The model under review builds one solid part; all positions refer to its coordinate system, in mm. Give positions to 0.01 mm unless a question says otherwise; leave off trailing zeros. Order: outer loops, then holes, each group sorted by start corner. A loop starts at its lowest first (then second) coordinate and runs counter-clockwise, first axis right, second up. Notation, with made-up numbers: (16.25, 66) - (31.25, 66) arc R34 cw to (31.25, 99) - close; hole circle Ø5 at (-19.75, -8.75). An arc over 180 degrees is marked (long way). Write item = value, one per line. Start each with the question number.
1. We need section B-B, the plane x = -3.81. Give the boundary of the cut face in (y, z).
2. We need section D-D, the plane z = -18.25. Give the boundary of the cut face in (x, y).
3. We need section C-C, the plane y = 0.2. State how many separate pieces and enclosed holes the cut face has, and give its area (3 significant figures).
4. Wall thickness on probe 1 along Z at (x, y) = (6, 0.25); probe 2 along Z at (x, y) = (-3.5, 0.2); probe 3 along X at (y, z) = (0.2, -19.25): over which ranges is each line inside the solid? List them lowest first.
5. We need section A-A, the plane x = 15.24. Give the boundary of the cut face in (y, z), and give its area (3 significant figures).
from build123d import *

# Parameters (mm, degrees)
SKETCH2_R               = 25.4
BOSS_EXTRUDE1_DEPTH     = 0.508
SKETCH3_R               = 1.016
CUT_EXTRUDE2_DEPTH      = 36.924616407
FILL_PATTERN1_OUTLINE_R = 1.016
FILL_PATTERN1_DEPTH     = 0.508
SKETCH7_W               = 63.5
SKETCH7_H               = 31.75
CUT_EXTRUDE5_DEPTH      = 36.924616407


# Read off the part's stored shape, not the designer's step: Fill Pattern1
with BuildPart() as part:
    # Sketch2 → Boss-Extrude1 (new body)
    with BuildSketch(Plane(origin=(0, 0, 0), x_dir=(1, 0, 0), z_dir=(0, 1, 0))):
        with Locations(Location((0, 0, 0), (0, 0, 270))):
            Circle(SKETCH2_R)
    extrude(amount=BOSS_EXTRUDE1_DEPTH)

    # Sketch3 → Cut-Extrude2 (cut, through all)
    with BuildSketch(Plane(origin=(0, 0.508, 0), x_dir=(1, 0, 0), z_dir=(0, 1, 0))):
        with Locations(Location((0, 0, 0), (0, 0, 270))):
            Circle(SKETCH3_R)
    extrude(amount=-CUT_EXTRUDE2_DEPTH, mode=Mode.SUBTRACT)

    # Fill Pattern1 outline → Fill Pattern1 (cut)
    with BuildSketch(Plane(origin=(0, 0, 0), x_dir=(1, 0, 0), z_dir=(0, 1, 0))):
        with Locations((20.955, -3.299556788)):
            Circle(FILL_PATTERN1_OUTLINE_R)
        with Locations((-11.43, -6.599113577)):
            Circle(FILL_PATTERN1_OUTLINE_R)
        with Locations((-13.335, -9.898670365)):
            Circle(FILL_PATTERN1_OUTLINE_R)
        with Locations((-15.24, -13.198227154)):
            Circle(FILL_PATTERN1_OUTLINE_R)
        with Locations((0, 19.797340731)):
            Circle(FILL_PATTERN1_OUTLINE_R)
        with Locations((-9.525, -3.299556788)):
            Circle(FILL_PATTERN1_OUTLINE_R)
        with Locations((-7.62, 0)):
            Circle(FILL_PATTERN1_OUTLINE_R)
        with Locations((-5.715, 3.299556788)):
            Circle(FILL_PATTERN1_OUTLINE_R)
        with Locations((-3.81, 6.599113577)):
            Circle(FILL_PATTERN1_OUTLINE_R)
        with Locations((-1.905, 16.497783942)):
            Circle(FILL_PATTERN1_OUTLINE_R)
        with Locations((-3.81, 13.198227154)):
            Circle(FILL_PATTERN1_OUTLINE_R)
        with Locations((-5.715, 9.898670365)):
            Circle(FILL_PATTERN1_OUTLINE_R)
        with Locations((-7.62, 6.599113577)):
            Circle(FILL_PATTERN1_OUTLINE_R)
        with Locations((-9.525, 3.299556788)):
            Circle(FILL_PATTERN1_OUTLINE_R)
        with Locations((-11.43, 0)):
            Circle(FILL_PATTERN1_OUTLINE_R)
        with Locations((-13.335, -3.299556788)):
            Circle(FILL_PATTERN1_OUTLINE_R)
        with Locations((-15.24, -6.599113577)):
            Circle(FILL_PATTERN1_OUTLINE_R)
        with Locations((7.62, 19.797340731)):
            Circle(FILL_PATTERN1_OUTLINE_R)
        with Locations((5.715, 16.497783942)):
            Circle(FILL_PATTERN1_OUTLINE_R)
        with Locations((3.81, 13.198227154)):
            Circle(FILL_PATTERN1_OUTLINE_R)
        with Locations((1.905, 9.898670365)):
            Circle(FILL_PATTERN1_OUTLINE_R)
        with Locations((0, 6.599113577)):
            Circle(FILL_PATTERN1_OUTLINE_R)
        with Locations((-1.905, 3.299556788)):
            Circle(FILL_PATTERN1_OUTLINE_R)
        with Locations((-3.81, 0)):
            Circle(FILL_PATTERN1_OUTLINE_R)
        with Locations((-5.715, -3.299556788)):
            Circle(FILL_PATTERN1_OUTLINE_R)
        with Locations((-7.62, -6.599113577)):
            Circle(FILL_PATTERN1_OUTLINE_R)
        with Locations((-9.525, -9.898670365)):
            Circle(FILL_PATTERN1_OUTLINE_R)
        with Locations((-11.43, -13.198227154)):
            Circle(FILL_PATTERN1_OUTLINE_R)
        with Locations((-13.335, -16.497783942)):
            Circle(FILL_PATTERN1_OUTLINE_R)
        with Locations((3.81, 19.797340731)):
            Circle(FILL_PATTERN1_OUTLINE_R)
        with Locations((1.905, 16.497783942)):
            Circle(FILL_PATTERN1_OUTLINE_R)
        with Locations((0, 13.198227154)):
            Circle(FILL_PATTERN1_OUTLINE_R)
        with Locations((-1.905, 9.898670365)):
            Circle(FILL_PATTERN1_OUTLINE_R)
        with Locations((-19.05, 0)):
            Circle(FILL_PATTERN1_OUTLINE_R)
        with Locations((-20.955, -3.299556788)):
            Circle(FILL_PATTERN1_OUTLINE_R)
        with Locations((-13.335, 16.497783942)):
            Circle(FILL_PATTERN1_OUTLINE_R)
        with Locations((-15.24, 13.198227154)):
            Circle(FILL_PATTERN1_OUTLINE_R)
        with Locations((-17.145, 9.898670365)):
            Circle(FILL_PATTERN1_OUTLINE_R)
        with Locations((-19.05, 6.599113577)):
            Circle(FILL_PATTERN1_OUTLINE_R)
        with Locations((-20.955, 3.299556788)):
            Circle(FILL_PATTERN1_OUTLINE_R)
        with Locations((-15.24, 0)):
            Circle(FILL_PATTERN1_OUTLINE_R)
        with Locations((-13.335, 3.299556788)):
            Circle(FILL_PATTERN1_OUTLINE_R)
        with Locations((-11.43, 6.599113577)):
            Circle(FILL_PATTERN1_OUTLINE_R)
        with Locations((-9.525, 9.898670365)):
            Circle(FILL_PATTERN1_OUTLINE_R)
        with Locations((-17.145, -9.898670365)):
            Circle(FILL_PATTERN1_OUTLINE_R)
        with Locations((-3.81, 19.797340731)):
            Circle(FILL_PATTERN1_OUTLINE_R)
        with Locations((-5.715, 16.497783942)):
            Circle(FILL_PATTERN1_OUTLINE_R)
        with Locations((-7.62, 13.198227154)):
            Circle(FILL_PATTERN1_OUTLINE_R)
        with Locations((-17.145, 3.299556788)):
            Circle(FILL_PATTERN1_OUTLINE_R)
        with Locations((-15.24, 6.599113577)):
            Circle(FILL_PATTERN1_OUTLINE_R)
        with Locations((-13.335, 9.898670365)):
            Circle(FILL_PATTERN1_OUTLINE_R)
        with Locations((-11.43, 13.198227154)):
            Circle(FILL_PATTERN1_OUTLINE_R)
        with Locations((-9.525, 16.497783942)):
            Circle(FILL_PATTERN1_OUTLINE_R)
        with Locations((-7.62, 19.797340731)):
            Circle(FILL_PATTERN1_OUTLINE_R)
        with Locations((-19.05, -6.599113577)):
            Circle(FILL_PATTERN1_OUTLINE_R)
        with Locations((-17.145, -3.299556788)):
            Circle(FILL_PATTERN1_OUTLINE_R)
        with Locations((3.81, -19.797340731)):
            Circle(FILL_PATTERN1_OUTLINE_R)
        with Locations((17.145, 9.898670365)):
            Circle(FILL_PATTERN1_OUTLINE_R)
        with Locations((15.24, 6.599113577)):
            Circle(FILL_PATTERN1_OUTLINE_R)
        with Locations((13.335, 3.299556788)):
            Circle(FILL_PATTERN1_OUTLINE_R)
        with Locations((5.715, -16.497783942)):
            Circle(FILL_PATTERN1_OUTLINE_R)
        with Locations((7.62, -13.198227154)):
            Circle(FILL_PATTERN1_OUTLINE_R)
        with Locations((9.525, -9.898670365)):
            Circle(FILL_PATTERN1_OUTLINE_R)
        with Locations((11.43, -6.599113577)):
            Circle(FILL_PATTERN1_OUTLINE_R)
        with Locations((3.81, -13.198227154)):
            Circle(FILL_PATTERN1_OUTLINE_R)
        with Locations((1.905, -16.497783942)):
            Circle(FILL_PATTERN1_OUTLINE_R)
        with Locations((0, -19.797340731)):
            Circle(FILL_PATTERN1_OUTLINE_R)
        with Locations((15.24, 13.198227154)):
            Circle(FILL_PATTERN1_OUTLINE_R)
        with Locations((5.715, -9.898670365)):
            Circle(FILL_PATTERN1_OUTLINE_R)
        with Locations((7.62, -6.599113577)):
            Circle(FILL_PATTERN1_OUTLINE_R)
        with Locations((9.525, -3.299556788)):
            Circle(FILL_PATTERN1_OUTLINE_R)
        with Locations((11.43, 0)):
            Circle(FILL_PATTERN1_OUTLINE_R)
        with Locations((15.24, -6.599113577)):
            Circle(FILL_PATTERN1_OUTLINE_R)
        with Locations((17.145, -3.299556788)):
            Circle(FILL_PATTERN1_OUTLINE_R)
        with Locations((19.05, 0)):
            Circle(FILL_PATTERN1_OUTLINE_R)
        with Locations((20.955, 3.299556788)):
            Circle(FILL_PATTERN1_OUTLINE_R)
        with Locations((13.335, -16.497783942)):
            Circle(FILL_PATTERN1_OUTLINE_R)
        with Locations((15.24, -13.198227154)):
            Circle(FILL_PATTERN1_OUTLINE_R)
        with Locations((17.145, -9.898670365)):
            Circle(FILL_PATTERN1_OUTLINE_R)
        with Locations((19.05, -6.599113577)):
            Circle(FILL_PATTERN1_OUTLINE_R)
        with Locations((13.335, -9.898670365)):
            Circle(FILL_PATTERN1_OUTLINE_R)
        with Locations((11.43, -13.198227154)):
            Circle(FILL_PATTERN1_OUTLINE_R)
        with Locations((9.525, -16.497783942)):
            Circle(FILL_PATTERN1_OUTLINE_R)
        with Locations((7.62, -19.797340731)):
            Circle(FILL_PATTERN1_OUTLINE_R)
        with Locations((19.05, 6.599113577)):
            Circle(FILL_PATTERN1_OUTLINE_R)
        with Locations((17.145, 3.299556788)):
            Circle(FILL_PATTERN1_OUTLINE_R)
        with Locations((15.24, 0)):
            Circle(FILL_PATTERN1_OUTLINE_R)
        with Locations((13.335, -3.299556788)):
            Circle(FILL_PATTERN1_OUTLINE_R)
        with Locations((7.62, 13.198227154)):
            Circle(FILL_PATTERN1_OUTLINE_R)
        with Locations((9.525, 16.497783942)):
            Circle(FILL_PATTERN1_OUTLINE_R)
        with Locations((-7.62, -19.797340731)):
            Circle(FILL_PATTERN1_OUTLINE_R)
        with Locations((-5.715, -16.497783942)):
            Circle(FILL_PATTERN1_OUTLINE_R)
        with Locations((-3.81, -13.198227154)):
            Circle(FILL_PATTERN1_OUTLINE_R)
        with Locations((-1.905, -9.898670365)):
            Circle(FILL_PATTERN1_OUTLINE_R)
        with Locations((0, -6.599113577)):
            Circle(FILL_PATTERN1_OUTLINE_R)
        with Locations((1.905, -3.299556788)):
            Circle(FILL_PATTERN1_OUTLINE_R)
        with Locations((5.715, 9.898670365)):
            Circle(FILL_PATTERN1_OUTLINE_R)
        with Locations((3.81, 6.599113577)):
            Circle(FILL_PATTERN1_OUTLINE_R)
        with Locations((1.905, 3.299556788)):
            Circle(FILL_PATTERN1_OUTLINE_R)
        with Locations((-1.905, -3.299556788)):
            Circle(FILL_PATTERN1_OUTLINE_R)
        with Locations((-3.81, -6.599113577)):
            Circle(FILL_PATTERN1_OUTLINE_R)
        with Locations((-5.715, -9.898670365)):
            Circle(FILL_PATTERN1_OUTLINE_R)
        with Locations((-7.62, -13.198227154)):
            Circle(FILL_PATTERN1_OUTLINE_R)
        with Locations((-9.525, -16.497783942)):
            Circle(FILL_PATTERN1_OUTLINE_R)
        with Locations((13.335, 9.898670365)):
            Circle(FILL_PATTERN1_OUTLINE_R)
        with Locations((11.43, 6.599113577)):
            Circle(FILL_PATTERN1_OUTLINE_R)
        with Locations((9.525, 3.299556788)):
            Circle(FILL_PATTERN1_OUTLINE_R)
        with Locations((7.62, 0)):
            Circle(FILL_PATTERN1_OUTLINE_R)
        with Locations((5.715, -3.299556788)):
            Circle(FILL_PATTERN1_OUTLINE_R)
        with Locations((3.81, -6.599113577)):
            Circle(FILL_PATTERN1_OUTLINE_R)
        with Locations((1.905, -9.898670365)):
            Circle(FILL_PATTERN1_OUTLINE_R)
        with Locations((0, -13.198227154)):
            Circle(FILL_PATTERN1_OUTLINE_R)
        with Locations((3.81, 0)):
            Circle(FILL_PATTERN1_OUTLINE_R)
        with Locations((5.715, 3.299556788)):
            Circle(FILL_PATTERN1_OUTLINE_R)
        with Locations((7.62, 6.599113577)):
            Circle(FILL_PATTERN1_OUTLINE_R)
        with Locations((9.525, 9.898670365)):
            Circle(FILL_PATTERN1_OUTLINE_R)
        with Locations((11.43, 13.198227154)):
            Circle(FILL_PATTERN1_OUTLINE_R)
        with Locations((13.335, 16.497783942)):
            Circle(FILL_PATTERN1_OUTLINE_R)
        with Locations((-3.81, -19.797340731)):
            Circle(FILL_PATTERN1_OUTLINE_R)
        with Locations((-1.905, -16.497783942)):
            Circle(FILL_PATTERN1_OUTLINE_R)
    extrude(amount=FILL_PATTERN1_DEPTH, mode=Mode.SUBTRACT)

    # Sketch7 → Cut-Extrude5 (cut, through all)
    with BuildSketch(Plane(origin=(0, 0.508, 0), x_dir=(1, 0, 0), z_dir=(0, 1, 0))):
        with Locations((0, -14.859)):
            Rectangle(SKETCH7_W, SKETCH7_H)
    extrude(amount=-CUT_EXTRUDE5_DEPTH, mode=Mode.SUBTRACT)


solid = part.part
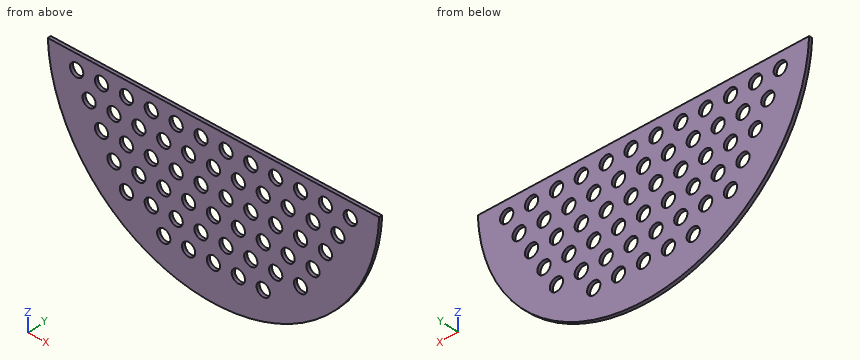
Model answer:
q1.outline = (0, -25.11) - (0.51, -25.11) - (0.51, -20.81) - (0, -20.81) - close; (0, -18.78) - (0.51, -18.78) - (0.51, -14.21) - (0, -14.21) - close; (0, -12.18) - (0.51, -12.18) - (0.51, -7.62) - (0, -7.62) - close; (0, -5.58) - (0.51, -5.58) - (0.51, -1.02) - (0, -1.02) - close
q2.outline = (-17.67, 0) - (17.67, 0) - (17.67, 0.51) - (-17.67, 0.51) - close
q3.separate_pieces = 1
q3.enclosed_holes = 55
q3.area = 783 mm2
q4.probe_1 = -24.68 to -17.47, -15.52 to -10.87, -8.92 to -4.27, -2.32 to -1.02
q4.probe_2 = -25.16 to -20.76, -18.83 to -14.17, -12.23 to -7.57, -5.63 to -1.02
q4.probe_3 = -16.57 to -8.48, -6.76 to -4.67, -2.95 to -0.86, 0.86 to 2.95, 4.67 to 6.76, 8.48 to 16.57
q5.outline = (0, -20.32) - (0.51, -20.32) - (0.51, -14.21) - (0, -14.21) - close; (0, -12.18) - (0.51, -12.18) - (0.51, -7.62) - (0, -7.62) - close; (0, -5.58) - (0.51, -5.58) - (0.51, -1.02) - (0, -1.02) - close
q5.area = 7.74 mm2
